from build123d import *

# Parameters (mm, degrees)
EXTRUDE_1_DEPTH          = 40
EXTRUDE_1_DEPTH_BACK     = 40
CUT_EXTRUDE_2_DEPTH      = 34
CUT_EXTRUDE_2_DEPTH_BACK = 34
CUT_EXTRUDE_3_DEPTH      = 38
CUT_EXTRUDE_3_DEPTH_BACK = 38
EXTRUDE_2_DEPTH          = 76
CUT_EXTRUDE_START        = -4
SKETCH_9_R               = 24
CUT_EXTRUDE_4_DEPTH      = 4
SKETCH_10_R              = 24
CUT_EXTRUDE_5_DEPTH      = 4
SKETCH_11_W              = 52
SKETCH_11_H              = 52
CUT_EXTRUDE_6_DEPTH      = 24
SKETCH_16_W              = 76
SKETCH_16_H              = 2
CUT_EXTRUDE_8_DEPTH      = 23.5
EXTRUDE_4_DEPTH          = 77.5
SKETCH_19_W              = 68
SKETCH_19_H              = 3
EXTRUDE_6_DEPTH          = 27
SKETCH_21_W              = 14
SKETCH_21_H              = 10
CUT_EXTRUDE_10_DEPTH     = 2
SKETCH_22_W              = 14
SKETCH_22_H              = 10
CUT_EXTRUDE_11_DEPTH     = 6
EXTRUDE_7_DEPTH          = 1.4
CUT_EXTRUDE_12_DEPTH     = 3.4
SKETCH_25_W              = 68
SKETCH_25_H              = 1
CUT_EXTRUDE_13_DEPTH     = 3.4
SKETCH_26_W              = 48
SKETCH_26_H              = 1.5
EXTRUDE_8_DEPTH          = 78
SKETCH_27_W              = 71
SKETCH_27_H              = 45
SKETCH_27_W_2            = 67
SKETCH_27_H_2            = 41
EXTRUDE_9_DEPTH          = 2.5
SKETCH_28_R              = 1.1
CUT_EXTRUDE_14_DEPTH     = 2
SKETCH_29_W              = 2
SKETCH_29_H              = 24
CUT_EXTRUDE_15_DEPTH     = 1


with BuildPart() as part:
    # Sketch 1 → Extrude 1 (new, two sides: drawn at the far end of the back side and taken through both)
    with BuildSketch(Plane(origin=(0, 0, 0), x_dir=(0, 0, -1), z_dir=(1, 0, 0)).offset(-EXTRUDE_1_DEPTH_BACK)):
        with BuildLine():
            Line((-75, 0), (-75, -15))
            Line((-75, -15), (-25, -26))
            Line((-25, -26), (-4.563728592, -26))
            Line((-4.563728592, -26), (25, -26))
            Line((25, -26), (75, -15))
            Line((75, -15), (75, 0))
            Line((75, 0), (24, 0))
            ThreePointArc((24, 0), (0, -24), (-24, 0))
            Line((-24, 0), (-75, 0))
        make_face()
    extrude(amount=EXTRUDE_1_DEPTH + EXTRUDE_1_DEPTH_BACK)

    # Sketch 3 → Cut-Extrude 2 (cut, two sides: drawn at the far end of the back side and taken through both)
    with BuildSketch(Plane(origin=(0, 0, 0), x_dir=(0, 0, -1), z_dir=(1, 0, 0)).offset(-CUT_EXTRUDE_2_DEPTH_BACK)):
        Polygon((26, 0), (73, 0), (73, -13.392171882), (23.878685446, -24), (-24.782599465, -24), (-73, -13.400590035), (-73, 0), (-26, 0), align=None)
    extrude(amount=CUT_EXTRUDE_2_DEPTH + CUT_EXTRUDE_2_DEPTH_BACK, mode=Mode.SUBTRACT)

    # Sketch 7 → Cut-Extrude 3 (cut, two sides: drawn at the far end of the back side and taken through both)
    with BuildSketch(Plane(origin=(0, 0, 0), x_dir=(0, 0, -1), z_dir=(1, 0, 0)).offset(-CUT_EXTRUDE_3_DEPTH_BACK)):
        Polygon((-26.2, 0), (26.2, 0), (73, 0), (73, -13.392171882), (23.963305429, -24), (10.509043724, -24), (-10.509043724, -24), (-24.782599465, -24), (-73, -14.042818852), (-73, 0), align=None)
    extrude(amount=CUT_EXTRUDE_3_DEPTH + CUT_EXTRUDE_3_DEPTH_BACK, mode=Mode.SUBTRACT)

    # Sketch 8 → Extrude 2 (add)
    with BuildSketch(Plane(origin=(-38, 0, 0), x_dir=(0, 0, -1), z_dir=(1, 0, 0))):
        with BuildLine():
            Line((-26, 0), (-22, 0))
            ThreePointArc((-22, 0), (0, -22), (22, 0))
            Line((22, 0), (26, 0))
            ThreePointArc((26, 0), (0, -26), (-26, 0))
        make_face()
    extrude(amount=EXTRUDE_2_DEPTH)

    # Sketch 9 → Cut-Extrude 4 (cut)
    with BuildSketch(Plane(origin=(38, 0, 0), x_dir=(0, 0, -1), z_dir=(1, 0, 0)).offset(CUT_EXTRUDE_START)):
        Circle(SKETCH_9_R)
    extrude(amount=CUT_EXTRUDE_4_DEPTH, mode=Mode.SUBTRACT)

    # Sketch 10 → Cut-Extrude 5 (cut)
    with BuildSketch(Plane.ZY.offset(38)):
        Circle(SKETCH_10_R)
    extrude(amount=-CUT_EXTRUDE_5_DEPTH, mode=Mode.SUBTRACT)

    # Sketch 11 → Cut-Extrude 6 (cut)
    with BuildSketch(Plane(origin=(0, 0, 0), x_dir=(1, 0, 0), z_dir=(0, 1, 0))):
        Rectangle(SKETCH_11_W, SKETCH_11_H)
    extrude(amount=-CUT_EXTRUDE_6_DEPTH, mode=Mode.SUBTRACT)

    # Sketch 16 → Cut-Extrude 8 (cut)
    with BuildSketch(Plane(origin=(0, 0, 0), x_dir=(1, 0, 0), z_dir=(0, 1, 0))):
        with Locations((0, -26)):
            Rectangle(SKETCH_16_W, SKETCH_16_H)
    extrude(amount=-CUT_EXTRUDE_8_DEPTH, mode=Mode.SUBTRACT)

    # Sketch 17 → Extrude 4 (add)
    with BuildSketch(Plane(origin=(-38, 0, 0), x_dir=(0, 0, -1), z_dir=(1, 0, 0))):
        Polygon((-73, -13.392171882), (-25.598256637, -13.392171882), (-25.598256637, -25.86838354), (-27.098256637, -25.53838354), (-27.098256637, -14.892171882), (-73, -14.892171882), align=None)
    extrude(amount=EXTRUDE_4_DEPTH)

    # Sketch 19 → Extrude 6 (add)
    with BuildSketch(Plane(origin=(0, 0, 0), x_dir=(1, 0, 0), z_dir=(0, 1, 0))):
        with Locations((0, -23.5)):
            Rectangle(SKETCH_19_W, SKETCH_19_H)
    extrude(amount=-EXTRUDE_6_DEPTH)

    # Sketch 21 → Cut-Extrude 10 (cut)
    with BuildSketch(Plane(origin=(0, -30.045784052, 6.610072491), x_dir=(1, 0, 0), z_dir=(0, -0.9766444667050901, 0.21486178267511963))):
        with Locations((-31, 63.025408263)):
            Rectangle(SKETCH_21_W, SKETCH_21_H)
    extrude(amount=-CUT_EXTRUDE_10_DEPTH, mode=Mode.SUBTRACT)

    # Sketch 22 → Cut-Extrude 11 (cut)
    with BuildSketch(Plane(origin=(0, -13.392171882, 0), x_dir=(1, 0, 0), z_dir=(0, 1, 0))):
        with Locations((-31, -68)):
            Rectangle(SKETCH_22_W, SKETCH_22_H)
    extrude(amount=-CUT_EXTRUDE_11_DEPTH, mode=Mode.SUBTRACT)

    # Sketch 23 → Extrude 7 (add)
    with BuildSketch(Plane.XZ.offset(14.892171882)):
        Polygon((-38, 63), (-24, 63), (-24, 73.046711067), (-22.5, 73.046711067), (-22.5, 64.14337403), (-22.5, 61.5), (-38, 61.5), align=None)
    extrude(amount=EXTRUDE_7_DEPTH)

    # Sketch 24 → Cut-Extrude 12 (cut)
    with BuildSketch(Plane(origin=(-22.5, 0, 0), x_dir=(0, 0, -1), z_dir=(1, 0, 0))):
        Polygon((-73.046711067, -15.429723565), (-69.126491444, -16.292171882), (-73.046711067, -16.292171882), align=None)
    extrude(amount=-CUT_EXTRUDE_12_DEPTH, mode=Mode.SUBTRACT)

    # Sketch 25 → Cut-Extrude 13 (cut)
    with BuildSketch(Plane(origin=(0, 0, 22), x_dir=(-1, 0, 0), z_dir=(0, 0, -1))):
        with Locations((0, -26.5)):
            Rectangle(SKETCH_25_W, SKETCH_25_H)
    extrude(amount=-CUT_EXTRUDE_13_DEPTH, mode=Mode.SUBTRACT)

    # Sketch 26 → Extrude 8 (add)
    with BuildSketch(Plane.ZY.offset(-38)):
        with Locations((-49, -12.642171882)):
            Rectangle(SKETCH_26_W, SKETCH_26_H)
    extrude(amount=EXTRUDE_8_DEPTH)

    # Sketch 27 → Extrude 9 (add)
    with BuildSketch(Plane(origin=(0, -11.892171882, 0), x_dir=(1, 0, 0), z_dir=(0, 1, 0))):
        with Locations((4.5, 52.5)):
            Rectangle(SKETCH_27_W, SKETCH_27_H)
        with Locations((4.5, 52.5)):
            Rectangle(SKETCH_27_W_2, SKETCH_27_H_2, mode=Mode.SUBTRACT)
    extrude(amount=EXTRUDE_9_DEPTH)

    # Sketch 28 → Cut-Extrude 14 (cut)
    with BuildSketch(Plane(origin=(0, -11.892171882, 0), x_dir=(1, 0, 0), z_dir=(0, 1, 0))):
        with Locations(Location((-26.5, 70.5, 0), (0, 0, 270))):
            Circle(SKETCH_28_R)
        with Locations(Location((-26.5, 34.5, 0), (0, 0, 270))):
            Circle(SKETCH_28_R)
        with Locations(Location((35.5, 70.5, 0), (0, 0, 270))):
            Circle(SKETCH_28_R)
        with Locations(Location((35.5, 34.5, 0), (0, 0, 270))):
            Circle(SKETCH_28_R)
    extrude(amount=-CUT_EXTRUDE_14_DEPTH, mode=Mode.SUBTRACT)

    # Sketch 29 → Cut-Extrude 15 (cut)
    with BuildSketch(Plane(origin=(0, -9.392171882, 0), x_dir=(1, 0, 0), z_dir=(0, 1, 0))):
        with Locations((-30, 51.5)):
            Rectangle(SKETCH_29_W, SKETCH_29_H)
    extrude(amount=-CUT_EXTRUDE_15_DEPTH, mode=Mode.SUBTRACT)


solid = part.part
Design review of the part built by this model. Coordinates are the model's own, in mm. A direction names the side the tool comes from. Coordinates: 2 decimals unless noted, no trailing zeros. Loops run counter-clockwise (first coordinate to the right, second up) from the corner with the lowest first, then second, coordinate; pieces in that order, holes last. Notation, with made-up numbers: (13.5, 50.5) -> (65.5, 50.5) arc R26 ccw to (65.5, 82.5) -> close; hole circle Ø7 at (74, 65.25). An arc over 180 degrees is marked (long way). Use a Markdown table: item, result. Add a question column.
Item 1: We need section B-B, the plane z = 0. Write out the cut boundary in (x, y), and give its area (3 significant figures).
Item 2: Wall thickness on L1, parallel to X at y = -12.25, z = -34.5; L2, parallel to Z at x = -8, y = -4.25; L3, parallel to X at y = -11.75, z = -51: over which ranges is each line inside the solid? List them lowest first. Write a range as from..to.
Item 3: We need section D-D, the plane x = 30.5. Count the separate pieces of the cut face and the enclosed holes in it, and give its area (3 significant figures).
Item 4: We need section C-C, the plane z = -58. Write out the cut boundary in (x, y), and give its area (3 significant figures).
Item 5: Machinability: for faces 4 (the flat face through (-1, -13.392, 50)), 5 (the flat face through (-1, -8, -75)), 6 (the flat face through (-34, -17, 24)), which of the approach directions +Z, -Z, +X, -X, +Y, -Y give a long, thin tool a straight path to every point of the face, cutting with its end or side? Answer none if there is none.
Item 6: Clearance check with flat-ended pins moving along their axes: P1, Ø2.5, axis at x = 35.5, z = -70.5, coming from the -Y side (3 decimals); P2, Ø9.5, axis at x = -8.5, y = -17.5, coming from the +Z side; P3, Ø6, axis at x = -28, z = 47, coming from the -Y side; P4, Ø0.6, axis at x = -29.5, z = -55, coming from the +Y side. State where each tip first meets the part, or that it passes through.
Item 7: We need section A-A, the plane x = 20. Write out the cut boundary in (y, z).
Item 8: The part is to be moulded in two halves that separate along X. For faces 1 (the flat face through (-31, -15, 63)), 2 (the flat face through (34, -17, 24)), 3 (the cylindrical face through (-30, -22, 0)), say which applies: +X half, -X half, draft (parallel to the pull), parting line (faces both ways), or undercut.
Numbers:
| question | item | result |
|---|---|---|
| 1 | outline | (-40, -26) -> (40, -26) -> (40, -24) -> (34, -24) -> (34, -22) -> (26, -22) -> (26, -24) -> (-26, -24) -> (-26, -22) -> (-34, -22) -> (-34, -24) -> (-40, -24) -> close |
| 1 | area | 192 mm^2 |
| 2 | L1 | x = -40..-27.6, -25.4..34.4, 36.6..40 |
| 2 | L2 | z = -75..-73, 22..25, 73..75 |
| 2 | L3 | x = -40..-38, -31..-29, 38..40 |
| 3 | separate pieces | 1 |
| 3 | enclosed holes | 2 |
| 3 | area | 815 mm^2 |
| 4 | outline | (-40, -18.74) -> (40, -18.74) -> (40, 0) -> (38, 0) -> (38, -11.89) -> (-29, -11.89) -> (-29, -10.39) -> (-31, -10.39) -> (-31, -11.89) -> (-38, -11.89) -> (-38, 0) -> (-40, 0) -> close; hole (-38, -16.64) -> (38, -16.64) -> (38, -13.39) -> (-38, -13.39) -> close |
| 4 | area | 352 mm^2 |
| 5 | face 4 | +Y |
| 5 | face 5 | -Z, +X, -X, +Y, -Y |
| 5 | face 6 | none |
| 6 | P1 | stops at y = -16.265 |
| 6 | P2 | stops at z = 75 |
| 6 | P3 | stops at y = -21.82 |
| 6 | P4 | stops at y = -10.39 |
| 7 | outline | (-26, -25) -> (-15, -75) -> (0, -75) -> (0, -73) -> (-11.89, -73) -> (-11.89, -32) -> (-9.39, -32) -> (-9.39, -30) -> (-11.89, -30) -> (-11.89, -25) -> (-13.39, -25) -> (-13.39, -73) -> (-23.56, -26) -> (-24, -26) -> (-24, 22) -> (0, 22) -> (0, 25) -> (-24, 25) -> (-24, 25.6) -> (-13.39, 25.6) -> (-13.39, 73) -> (0, 73) -> (0, 75) -> (-15, 75) -> (-26, 25) -> close; hole (-23.52, 27.1) -> (-14.89, 27.1) -> (-14.89, 68.89) -> close |
| 8 | face 1 | undercut |
| 8 | face 2 | undercut |
| 8 | face 3 | draft |
